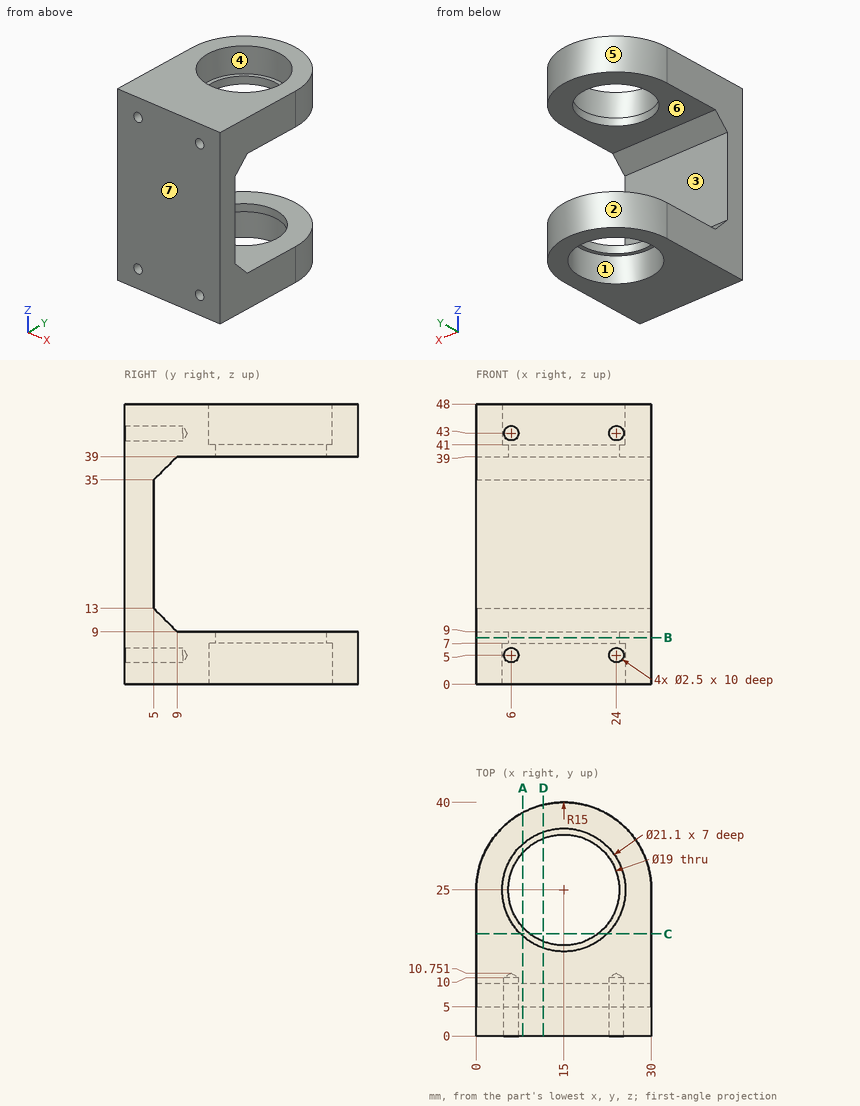
Design review of the part shown in the three views and the two pictorial views. Dimensions are in mm from the part's minimum x, y and z. A direction names the side the tool comes from. Give positions to 0.01 mm unless a question says otherwise; leave off trailing zeros. Loops run counter-clockwise (first coordinate to the right, second up) from the corner with the lowest first, then second, coordinate; pieces in that order, holes last. Notation, with made-up numbers: (59.25, 1.25) -> (97.25, 1.25) arc R23 ccw to (97.25, 13.25) -> close; hole circle Ø11 at (-0.75, -13). An arc over 180 degrees is marked (long way). Put each result on its own line as item: value. Start each with the question number.
1. We need section D-D on x = 11.5. State the section outline as (y, z) points.
2. Mouldability with a two-part tool opening along Y and no side actions: class the marked faces 4, 5, 6 and 7 as released by +Y, released by -Y, zero draft, split by the parting line, or undercut.
3. Wall thickness on probe 1 along Z at (x, y) = (24, 2.25); probe 2 along Z at (x, y) = (18.5, 14.5); probe 3 along Z at (x, y) = (24, 5.25): over which ranges is each line inside the solid? List them lowest first.
4. Clearance check with flat-ended pins moving along their axes: P1, Ø1.5, axis at x = 24, z = 5, coming from the +Y side; P2, Ø11, axis at x = 19, z = 29, coming from the +Y side; P3, Ø17, axis at x = 11.5, y = 24, coming from the -Z side; P4, Ø2, axis at x = 6, z = 5, coming from the +Y side. State where each tip first meets the part, or that it passes through.
5. We need section A-A on x = 8. State the section outline as (y, z) points, then the cut area to 3 significant figures.
6. For the marked faces 1, 2 and 3, list the 3-axis set-ups (+Z, -Z, +X, -X, +Y, -Y) from which the entire face can be reached by the end or side of a thin tool; tool diameter is ignored.
7. We need section C-C on y = 17.5. State the section outline as (x, z) points, then the cut area to 3 significant figures.
8. We need section B-B on z = 8. State the section outline as (x, y) points.
Determined:
1. outline: (0, 0) -> (15.05, 0) -> (15.05, 7) -> (16.17, 7) -> (16.17, 9) -> (9, 9) -> (5, 13) -> (5, 35) -> (9, 39) -> (16.17, 39) -> (16.17, 41) -> (15.05, 41) -> (15.05, 48) -> (0, 48) -> close; (33.83, 7) -> (34.95, 7) -> (34.95, 0) -> (39.59, 0) -> (39.59, 9) -> (33.83, 9) -> close; (33.83, 39) -> (39.59, 39) -> (39.59, 48) -> (34.95, 48) -> (34.95, 41) -> (33.83, 41) -> close
2. face 4: undercut
2. face 5: released by +Y
2. face 6: zero draft
2. face 7: released by -Y
3. probe 1: 0 to 3.75, 6.25 to 41.75, 44.25 to 48
3. probe 2: 0 to 9, 39 to 48
3. probe 3: 0 to 3.75, 6.25 to 12.75, 35.25 to 41.75, 44.25 to 48
4. P1: y = 37.53
4. P2: y = 5
4. P3: z = 0
4. P4: y = 37.69
5. outline: (0, 0) -> (17.11, 0) -> (17.11, 7) -> (18.58, 7) -> (18.58, 9) -> (9, 9) -> (5, 13) -> (5, 35) -> (9, 39) -> (18.58, 39) -> (18.58, 41) -> (17.11, 41) -> (17.11, 48) -> (0, 48) -> close; (31.42, 7) -> (32.89, 7) -> (32.89, 0) -> (38.27, 0) -> (38.27, 9) -> (31.42, 9) -> close; (31.42, 39) -> (38.27, 39) -> (38.27, 48) -> (32.89, 48) -> (32.89, 41) -> (31.42, 41) -> close
5. area: 582 mm^2
6. face 1: -Z
6. face 2: +Z, -Z, +Y
6. face 3: +X, -X, +Y
7. outline: (0, 0) -> (7.58, 0) -> (7.58, 7) -> (9.17, 7) -> (9.17, 9) -> (0, 9) -> close; (0, 39) -> (9.17, 39) -> (9.17, 41) -> (7.58, 41) -> (7.58, 48) -> (0, 48) -> close; (20.83, 7) -> (22.42, 7) -> (22.42, 0) -> (30, 0) -> (30, 9) -> (20.83, 9) -> close; (20.83, 39) -> (30, 39) -> (30, 48) -> (22.42, 48) -> (22.42, 41) -> (20.83, 41) -> close
7. area: 286 mm^2
8. outline: (0, 0) -> (30, 0) -> (30, 25) arc R15 ccw to (0, 25) -> close; hole circle Ø19 at (15, 25)
